Design review of the part shown in the three views and the two pictorial views. Dimensions are in mm from the part's minimum x, y and z. A direction names the side the tool comes from. Coordinates: 2 decimals unless noted, no trailing zeros. Loops run counter-clockwise (first coordinate to the right, second up) from the corner with the lowest first, then second, coordinate; pieces in that order, holes last.
Q1. Wall thickness on probe 1 along Z at (x, y) = (22.5, 13); probe 2 along X at (y, z) = (42, 84.5) (1 decimal); probe 3 along Z at (x, y) = (69, 34): over which ranges is each line inside the solid? List them lowest first.
Q2. For P1, Ø6, axis at x = 39.5, z = 60.5, coming from the -Y side; P2, Ø12, axis at y = 32.5, z = 70, coming from the +X side (1 decimal); P3, Ø2, axis at x = 54.5, y = 57, coming from the +Z side; P4, Ø2, axis at y = 23, z = 23, coming from the +X side, all flat-tipped, find the tip position at first contact; note any pin that passes through.
Q3. Add section B-B on x = 67. Give the boundary of the cut face in (y, z).
Q4. Add section D-D on y = 65.5. Give the boundary of the cut face in (x, z).
Q5. Add section A-A on y = 14.5. Give the boundary of the cut face in (x, z).
Q6. Add section C-C on z = 79. Give the boundary of the cut face in (x, y) (1 decimal), and give its area (3 significant figures).
Q7. Machinability: for the marked faces 1, 2 and 3, which of the approach directions +Z, -Z, +X, -X, +Y, -Y give a long, thin tool a straight path to every point of the face, cutting with its end or side? Answer none if there is none.
Q8. Draft analysis for pull direction Z (two halves, no side actions). For the marked faces 4, 5, 6 and 7, state which applies: released by +Z, released by -Z, zero draft, split by the parting line, or undercut.
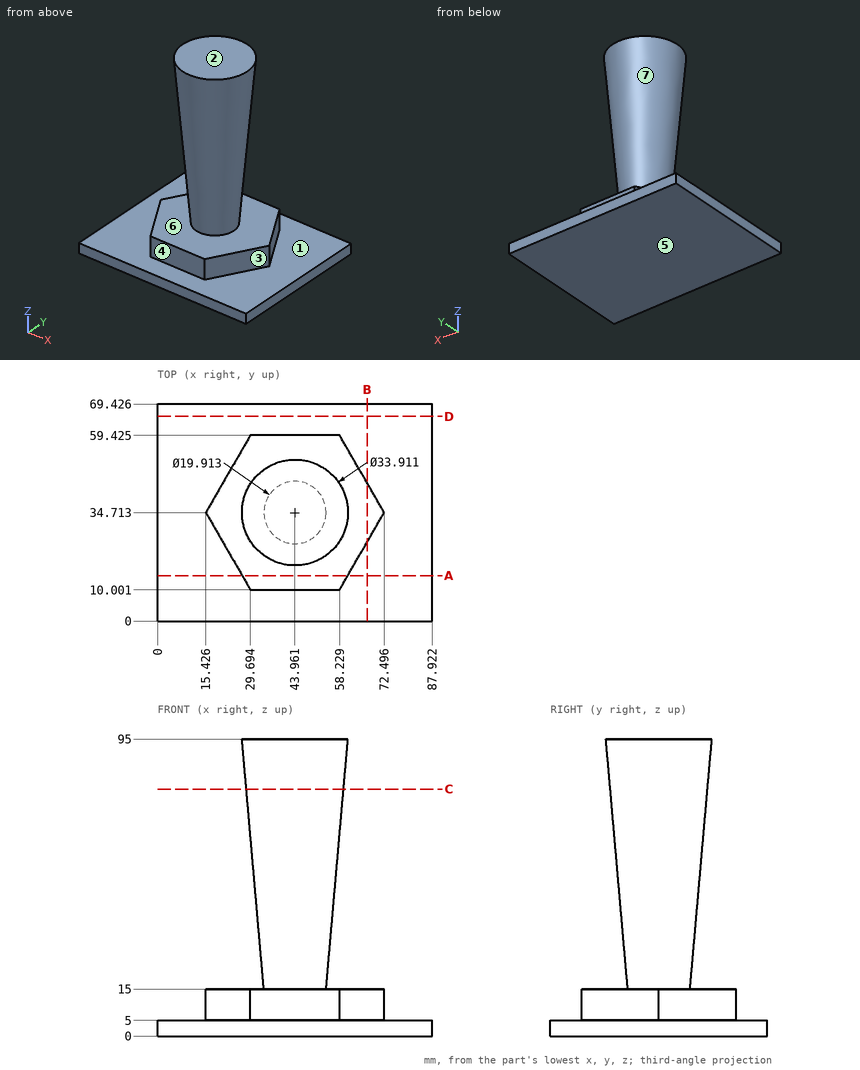
Entries:
1. probe 1: z = 0 to 5
1. probe 2: x = 29.7 to 58.2
1. probe 3: z = 0 to 15
2. P1: stops at y = 20.77
2. P2: stops at x = 59.2
2. P3: stops at z = 15
2. P4: passes through
3. outline: (0, 0) - (69.43, 0) - (69.43, 5) - (44.23, 5) - (44.23, 15) - (25.19, 15) - (25.19, 5) - (0, 5) - close
4. outline: (0, 0) - (87.92, 0) - (87.92, 5) - (0, 5) - close
5. outline: (0, 0) - (87.92, 0) - (87.92, 5) - (60.83, 5) - (60.83, 15) - (27.1, 15) - (27.1, 5) - (0, 5) - close
6. outline: circle Ø31.1 at (44, 34.7)
6. area: 760 mm2
7. face 1: +Z
7. face 2: +Z, +X, -X, +Y, -Y
7. face 3: +Z, +X, -Y
8. face 4: zero draft
8. face 5: released by -Z
8. face 6: undercut
8. face 7: undercut
